Design review of the part built by this model. Coordinates are the model's own, in mm. Coordinates: 2 decimals unless noted, no trailing zeros. Loops run counter-clockwise (first coordinate to the right, second up) from the corner with the lowest first, then second, coordinate; pieces in that order, holes last.
from build123d import *

# Parameters (mm, degrees)
PAD087_DEPTH    = 3
POCKET016_DEPTH = 3.001
CHAMFER060_SIZE = 1
SKETCH179_R     = 1.6
POCKET025_DEPTH = 3.001
SKETCH180_R     = 1.6
SKETCH180_W     = 10
SKETCH180_H     = 3
POCKET026_DEPTH = 3.001
POCKET027_DEPTH = 3.001


with BuildPart() as part:
    # Sketch160 → Pad087 (new body)
    with BuildSketch(Plane(origin=(0, 0, 0), x_dir=(-1, 0, 0), z_dir=(0, 1, 0))):
        Polygon((-40, 310), (-30, 310), (-30, 320), (30, 320), (30, 310), (40, 310), (40, 120), (-40, 120), align=None)
    extrude(amount=PAD087_DEPTH)

    # Sketch161 → Pocket016 (cut, through all)
    with BuildSketch(Plane(origin=(0, 0, 0), x_dir=(-1, 0, 0), z_dir=(0, 1, 0))):
        with BuildLine():
            ThreePointArc((-40, 294), (-44, 290), (-40, 286))
            Line((-40, 286), (-35, 286))
            ThreePointArc((-35, 286), (-31, 290), (-35, 294))
            Line((-35, 294), (-40, 294))
        make_face()
        with BuildLine():
            ThreePointArc((-40, 144), (-44, 140), (-40, 136))
            Line((-40, 136), (-35, 136))
            ThreePointArc((-35, 136), (-31, 140), (-35, 144))
            Line((-35, 144), (-40, 144))
        make_face()
        with BuildLine():
            ThreePointArc((40, 136), (44, 140), (40, 144))
            Line((40, 144), (35, 144))
            ThreePointArc((35, 144), (31, 140), (35, 136))
            Line((35, 136), (40, 136))
        make_face()
        with BuildLine():
            ThreePointArc((40, 191), (44, 195), (40, 199))
            Line((40, 199), (35, 199))
            ThreePointArc((35, 199), (31, 195), (35, 191))
            Line((35, 191), (40, 191))
        make_face()
    extrude(amount=POCKET016_DEPTH, mode=Mode.SUBTRACT)

    # Chamfer060
    chamfer060_edges = [part.edges().sort_by_distance(p)[0] for p in [
        (40, 1.5, 310),
        (30, 1.5, 320),
        (40, 1.5, 294),
        (40, 1.5, 286),
        (-40, 1.5, 310),
        (-30, 1.5, 320),
        (40, 1.5, 144),
        (40, 1.5, 136),
        (40, 1.5, 120),
        (-40, 1.5, 120),
        (-40, 1.5, 136),
        (-40, 1.5, 144),
        (-40, 1.5, 191),
        (-40, 1.5, 199),
    ]]
    chamfer(chamfer060_edges, length=CHAMFER060_SIZE)

    # Sketch179 (on Face5 of Chamfer060) → Pocket025 (cut, through all)
    with BuildSketch(Plane(origin=(0, 3, 0), x_dir=(1, 0, 0), z_dir=(0, 1, 0))):
        with Locations((-25.769897, -208.69686)):
            Circle(SKETCH179_R)
        with Locations((23.730103, -208.69686)):
            Circle(SKETCH179_R)
        with Locations((23.730103, -300.69686)):
            Circle(SKETCH179_R)
        with Locations((-25.769897, -300.69686)):
            Circle(SKETCH179_R)
        Polygon((26.480103, -297.94686), (-28.519897, -297.94686), (-28.519897, -260.94686), (-30.019897, -260.94686), (-30.019897, -253.44686), (-28.519897, -253.44686), (-28.519897, -211.44686), (26.480103, -211.44686), (26.480103, -253.44686), (27.980103, -253.44686), (27.980103, -260.94686), (26.480103, -260.94686), align=None)
    extrude(amount=-POCKET025_DEPTH, mode=Mode.SUBTRACT)

    # Sketch180 (on Face5 of Pocket025) → Pocket026 (cut, through all)
    with BuildSketch(Plane(origin=(0, 3, 0), x_dir=(-1, 0, 0), z_dir=(0, 1, 0))):
        with Locations((23.62, 163.37)):
            Circle(SKETCH180_R)
        with Locations((3.62, 163.37)):
            Circle(SKETCH180_R)
        with Locations((13.62, 163.37)):
            Rectangle(SKETCH180_W, SKETCH180_H)
    extrude(amount=-POCKET026_DEPTH, mode=Mode.SUBTRACT)

    # Sketch182 → Pocket027 (cut, through all)
    with BuildSketch(Plane.XZ):
        with BuildLine():
            ThreePointArc((-21.019897, 209.69686), (-23.519897, 207.19686), (-21.019897, 204.69686))
            Line((-21.019897, 204.69686), (18.980103, 204.69686))
            ThreePointArc((18.980103, 204.69686), (21.480103, 207.19686), (18.980103, 209.69686))
            Line((18.980103, 209.69686), (-21.019897, 209.69686))
        make_face()
    extrude(amount=-POCKET027_DEPTH, mode=Mode.SUBTRACT)


with BuildPart() as part_1:
    # Body076 placement: moved
    add(part.part.moved(Location((0, 75, 0))))


solid = part_1.part
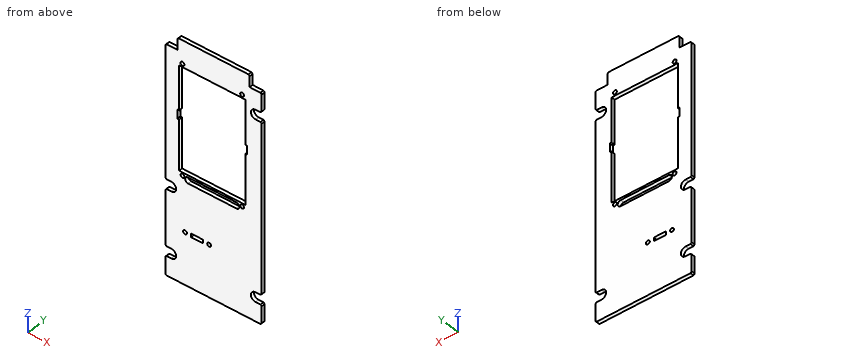
Q1. Take a section at C-C, the plane z = 289. Write out the cut boundary in (x, y), then the cut area to 3 significant figures.
Q2. Take a section at A-A, the plane z = 244.5. Write out the cut boundary in (x, y), then the cut area to 3 significant figures.
Q3. Take a section at B-B, the plane x = -14. Write out the cut boundary in (y, z), then the cut area to 4 significant figures.
Q4. Clearance check with flat-ended pins moving along their axes: pin 1 Ø3 at (x, z) = (23.73, 208.7) entering from +Y; pin 2 Ø1.5 at (x, y) = (-37.5, 76) entering from +Z. State where each tip first meets the part, or that it passes through.
Q5. Take a section at D-D, the plane y = 77.5. Give the number of separate pieces and of enclosed holes in the cut face, then the cut area to 3 significant figures.
Q6. For line 1 (Z direction, x = -3.62, y = 76); line 2 (Z direction, x = -19, y = 76.75); line 3 (X direction, y = 77.05, z = 163.37), list the stretches that pass through material, from the lowest coordinate up.
Entries:
1. outline: (-40, 75) - (-28.52, 75) - (-28.52, 78) - (-40, 78) - close; (26.48, 75) - (31.13, 75) - (31.13, 78) - (26.48, 78) - close
1. area: 48.4 mm2
2. outline: (-40, 75) - (-28.52, 75) - (-28.52, 78) - (-40, 78) - close; (26.48, 75) - (40, 75) - (40, 78) - (26.48, 78) - close
2. area: 75.0 mm2
3. outline: (75, 120) - (78, 120) - (78, 161.87) - (75, 161.87) - close; (75, 164.87) - (78, 164.87) - (78, 204.7) - (75, 204.7) - close; (75, 209.7) - (78, 209.7) - (78, 211.45) - (75, 211.45) - close; (75, 297.95) - (78, 297.95) - (78, 320) - (75, 320) - close
3. area: 316.5 mm2
4. pin 1: passes through
4. pin 2: stops at z = 310
5. separate pieces: 1
5. enclosed holes: 9
5. area: 10,500 mm2
6. line 1: z = 120 to 161.77, 164.97 to 204.7, 209.7 to 211.45, 297.95 to 320
6. line 2: z = 120 to 204.7, 209.7 to 211.45, 297.95 to 320
6. line 3: x = -40 to -25.22, -22.02 to -18.62, -8.62 to -5.22, -2.02 to 40
